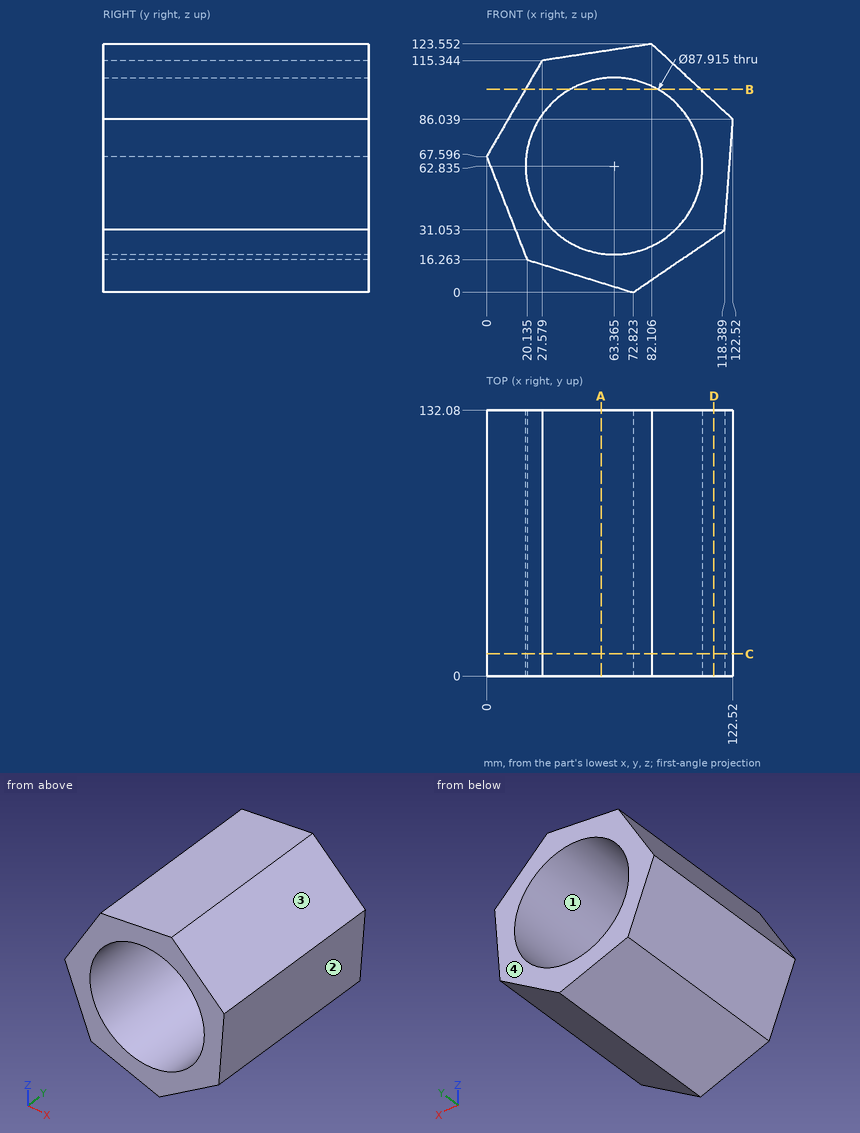
Can you work these out from the drawing? Everything is in mm from the part's minimum corner. Coordinates: 2 decimals unless noted, no trailing zeros. Loops run counter-clockwise (first coordinate to the right, second up) from the corner with the lowest first, then second, coordinate; pieces in that order, holes last.
1) Imagine slicing it at A-A (x = 57). List the corners of the cut face in (y, z) for me (1 decimal).
Reported:
outline: (0, 4.9) - (132.1, 4.9) - (132.1, 19.3) - (0, 19.3) - close; (0, 106.3) - (132.1, 106.3) - (132.1, 119.8) - (0, 119.8) - close
2) Please list where these lines run through material, in increasing order: line 1 along Z through (x, y) = (31, 45.5); line 2 along X through (y, z) = (84, 55.5) (1 decimal); line 3 along Z through (x, y) = (88, 7) (1 decimal).
Reported:
line 1: z = 12.91 to 33.09, 92.58 to 115.86
line 2: x = 4.7 to 20, 106.7 to 120.2
line 3: z = 10.3 to 26.4, 99.2 to 118.1
3) Imagine slicing it at B-B (z = 101). List the corners of the cut face in (x, y) for me (1 decimal).
Reported:
outline: (19.3, 0) - (41.6, 0) - (41.6, 132.1) - (19.3, 132.1) - close; (85.2, 0) - (106.4, 0) - (106.4, 132.1) - (85.2, 132.1) - close
4) Will these pins go through, and if not, where does the flat tip stop? pin 1 Ø8 at (x, y) = (54.5, 97.5) entering from -Z; pin 2 Ø3 at (x, y) = (21.5, 85) entering from -Z; pin 3 Ø12 at (x, y) = (30, 87.5) entering from -Z.
Reported:
pin 1: stops at z = 4.42
pin 2: stops at z = 15.38
pin 3: stops at z = 11.37
5) Imagine slicing it at D-D (x = 113). List the corners of the cut face in (y, z) for me (1 decimal).
Reported:
outline: (0, 27.4) - (132.1, 27.4) - (132.1, 94.9) - (0, 94.9) - close
6) Imagine slicing it at C-C (y = 11). List the corners of the cut face in (x, z) for me (1 decimal), and give its area (3 significant figures).
Reported:
outline: (0, 67.6) - (20.1, 16.3) - (72.8, 0) - (118.4, 31.1) - (122.5, 86) - (82.1, 123.6) - (27.6, 115.3) - close; hole circle Ø87.9 at (63.4, 62.8)
area: 4,980 mm2
7) Thinking about a two-plate mould opening in Z: for the marked faces 1, 2, 3 and 4, which applies, released by +Z, released by -Z, zero draft, split by the parting line, or undercut?
Reported:
face 1: undercut
face 2: released by -Z
face 3: released by +Z
face 4: zero draft
